Geometry check sheet. Reference: the model listing, model coordinates, mm. Face numbers are marked on the shaded views. A direction names the side the tool comes from. Coordinates: 2 decimals unless noted, no trailing zeros. Write each loop counter-clockwise with the first axis right and the second up, starting at its lowest first coordinate (ties: lowest second). Pieces come first, ordered by that corner, then holes. Notation, with made-up numbers: (81, 50.5) -> (90, 50.5) arc R11 cw to (90, 63.5) -> close; hole circle Ø5 at (-10.5, -10). An arc over 180 degrees is marked (long way). Answer in a Markdown table with one row per item. Add a question column.
1. Set-up check for the marked faces 1, 2, 3 and 4: record each of +Z, -Z, +X, -X, +Y, -Y from which the full face is reachable in a straight line by a thin tool's end or side.
2. Cross-section at B-B on x = -3.75. Record the cut outline in (y, z).
3. Scan lines: L1, parallel to Z at x = 6.5, y = 11; L2, parallel to X at y = 108, z = 2.5. Record each from-to range of solid material in increasing order. Write a range as from..to.
4. Depth check by flat-ended pin: P1, Ø8, axis at y = 91, z = 0.5, coming from the +X side; P2, Ø1.1, axis at x = 7, z = 2, coming from the +Y side; P3, Ø4, axis at x = 2.5, y = 100, coming from the -Z side; P4, Ø8, axis at y = 57.5, z = -6.5, coming from the -X side. Enter the tip coordinate at first touch or a pass-through.
5. Cross-section at A-A on z = 0. Record the cut outline in (x, y), and give its area (3 significant figures).
6. Cross-section at C-C on y = 104. Record the cut outline in (x, z), and give its area (3 significant figures).
7. Cross-section at D-D on x = 2. Record the cut outline in (y, z).
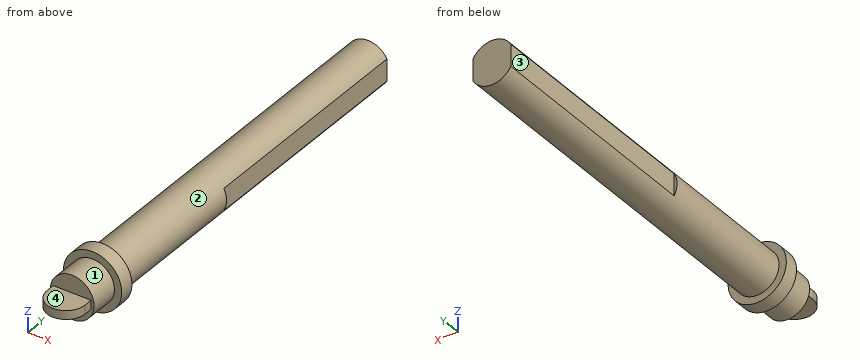
```python
from build123d import *

# Parameters (mm, degrees)
SKETCH3_R                = 7.5
BOSS_EXTRUDE1_DEPTH      = 130
SKETCH4_R                = 10
BOSS_EXTRUDE2_DEPTH      = 5
BOSS_EXTRUDE3_START      = 10
SKETCH5_R                = 7.5
BOSS_EXTRUDE3_DEPTH      = 10
BOSS_EXTRUDE4_DEPTH      = 1.5
BOSS_EXTRUDE4_DEPTH_BACK = 1.5
CUT_EXTRUDE1_START       = -80
CUT_EXTRUDE1_DEPTH       = 80


with BuildPart() as part:
    # Sketch3 → Boss-Extrude1 (new body)
    with BuildSketch(Plane(origin=(0, 0, 0), x_dir=(1, 0, 0), z_dir=(0, 1, 0))):
        with Locations(Location((0, 0, 0), (0, 0, 270))):
            Circle(SKETCH3_R)
    extrude(amount=BOSS_EXTRUDE1_DEPTH)

    # Sketch4 → Boss-Extrude2 (add)
    with BuildSketch(Plane.XZ):
        with Locations(Location((0, 0, 0), (0, 0, 270))):
            Circle(SKETCH4_R)
    extrude(amount=BOSS_EXTRUDE2_DEPTH)

    # Sketch5 → Boss-Extrude3 (add)
    with BuildSketch(Plane.XZ.offset(5).offset(BOSS_EXTRUDE3_START)):
        with Locations(Location((0, 0, 0), (0, 0, 90))):
            Circle(SKETCH5_R)
    extrude(amount=-BOSS_EXTRUDE3_DEPTH)

    # Sketch7 → Boss-Extrude4 (add, two sides: drawn at the far end of the back side and taken through both)
    with BuildSketch(Plane.XY.offset(-BOSS_EXTRUDE4_DEPTH_BACK)):
        with BuildLine():
            Line((-6.5, -15), (6.5, -15))
            Line((6.5, -15), (6.5, -18))
            ThreePointArc((6.5, -18), (0, -24.5), (-6.5, -18))
            Line((-6.5, -18), (-6.5, -15))
        make_face()
    extrude(amount=BOSS_EXTRUDE4_DEPTH + BOSS_EXTRUDE4_DEPTH_BACK)

    # Sketch8 → Cut-Extrude1 (cut)
    with BuildSketch(Plane(origin=(0, 130, 0), x_dir=(1, 0, 0), z_dir=(0, 1, 0)).offset(CUT_EXTRUDE1_START)):
        with BuildLine():
            Line((6.5, 3.741657387), (6.5, -3.741657387))
            ThreePointArc((6.5, -3.741657387), (7.5, 0), (6.5, 3.741657387))
        make_face()
        with BuildLine():
            Line((-6.5, 3.741657387), (-6.5, -3.741657387))
            ThreePointArc((-6.5, -3.741657387), (-7.5, 0), (-6.5, 3.741657387))
        make_face()
    extrude(amount=CUT_EXTRUDE1_DEPTH, mode=Mode.SUBTRACT)


solid = part.part
```
Results found:
| question | item | result |
|---|---|---|
| 1 | face 1 | -Y |
| 1 | face 2 | +Y |
| 1 | face 3 | +Z, -Z, -X, +Y |
| 1 | face 4 | +Z, +X, -X, -Y |
| 2 | outline | (-23.31, -1.5) -> (-15, -1.5) -> (-15, -6.5) -> (-5, -6.5) -> (-5, -9.27) -> (0, -9.27) -> (0, -6.5) -> (130, -6.5) -> (130, 6.5) -> (0, 6.5) -> (0, 9.27) -> (-5, 9.27) -> (-5, 6.5) -> (-15, 6.5) -> (-15, 1.5) -> (-23.31, 1.5) -> close |
| 3 | L1 | z = -3.74..3.74 |
| 3 | L2 | x = -6.5..6.5 |
| 4 | P1 | stops at x = 6.5 |
| 4 | P2 | stops at y = 130 |
| 4 | P3 | stops at z = -7.48 |
| 4 | P4 | stops at x = -6.5 |
| 5 | outline | (-10, -5) -> (-7.5, -5) -> (-7.5, -15) -> (-6.5, -15) -> (-6.5, -18) arc R6.5 ccw to (6.5, -18) -> (6.5, -15) -> (7.5, -15) -> (7.5, -5) -> (10, -5) -> (10, 0) -> (7.5, 0) -> (7.5, 50) -> (6.5, 50) -> (6.5, 130) -> (-6.5, 130) -> (-6.5, 50) -> (-7.5, 50) -> (-7.5, 0) -> (-10, 0) -> close |
| 5 | area | 2,150 mm^2 |
| 6 | outline | (-6.5, -3.74) arc R7.5 ccw to (6.5, -3.74) -> (6.5, 3.74) arc R7.5 ccw to (-6.5, 3.74) -> close |
| 6 | area | 167 mm^2 |
| 7 | outline | (-24.18, -1.5) -> (-15, -1.5) -> (-15, -7.23) -> (-5, -7.23) -> (-5, -9.8) -> (0, -9.8) -> (0, -7.23) -> (130, -7.23) -> (130, 7.23) -> (0, 7.23) -> (0, 9.8) -> (-5, 9.8) -> (-5, 7.23) -> (-15, 7.23) -> (-15, 1.5) -> (-24.18, 1.5) -> close |
